The listing builds one solid part. Answer for the finished solid, in the listing's coordinates (mm). Face numbers are marked on the shaded views. Round coordinates to 2 decimals unless told otherwise and drop trailing zeros. Write each loop counter-clockwise with the first axis right and the second up, starting at its lowest first coordinate (ties: lowest second). Pieces come first, ordered by that corner, then holes.
(1) The mould has two halves that part along Y. Classify the marked faces 1, 2 and 3: +Y half, -Y half, draft (parallel to the pull), parting line (faces both ways), or undercut.
(2) A cutting plane is placed at C-C, the plane z = 0. Give the number of separate pieces and of enclosed holes in the cut face, and give its area (3 significant figures).
(3) A cutting plane is placed at D-D, the plane y = 65. Give the vertices of the cut face in (x, z), and give its area (3 significant figures).
(4) A cutting plane is placed at B-B, the plane x = -15.5. Give the vertices of the cut face in (y, z), and give its area (3 significant figures).
(5) Each of these flat-tipped pins is pushed along its axis until it touches: pin 1 Ø10 at (y, z) = (-7.5, -5) entering from -X; pin 2 Ø1.5 at (y, z) = (110.5, -10) entering from +X; pin 3 Ø5 at (y, z) = (2.5, -5.5) entering from +X. Where does it stop, or does it pass through?
(6) A cutting plane is placed at A-A, the plane x = -102. Give the vertices of the cut face in (y, z).
(7) Find the intervals of material crossed by probe 1 along Y at (x, z) = (-43.5, -7.5); probe 2 along Y at (x, z) = (-133, -2); probe 3 along Z at (x, y) = (-125, -23.55), in increasing order.
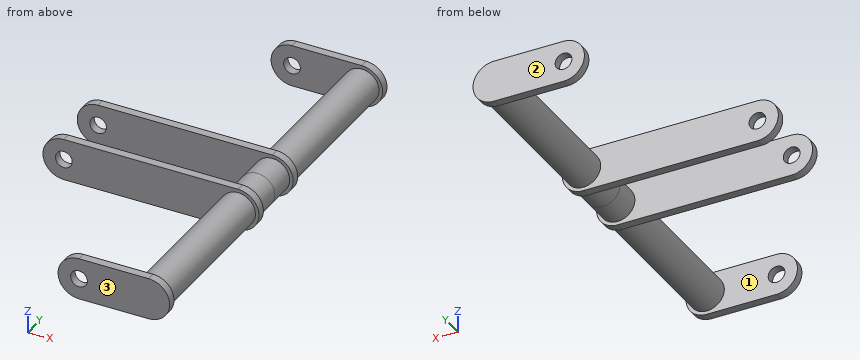
from build123d import *

# Parameters (mm, degrees)
F1_R     = 6
F1_R_2   = 12.5
F2_DEPTH = 6
F3_DEPTH = 140
F5_R     = 6
F6_DEPTH = 6


with BuildPart() as f2:
    # F1 (on offset) → F2 (new body)
    with BuildSketch(Plane.XZ.offset(140)):
        with BuildLine():
            Line((-50, -15), (0, -15))
            ThreePointArc((0, -15), (15, 0), (0, 15))
            Line((0, 15), (-50, 15))
            ThreePointArc((-50, 15), (-65, 0), (-50, -15))
        make_face()
        with Locations((-50, 0)):
            Circle(F1_R, mode=Mode.SUBTRACT)
        Circle(F1_R_2, mode=Mode.SUBTRACT)
        Circle(F1_R_2)
        Circle(F1_R, mode=Mode.SUBTRACT)
        Circle(F1_R)
    extrude(amount=F2_DEPTH)

    # F1 (on offset) → F3 (join, through all)
    with BuildSketch(Plane.XZ.offset(140)):
        Circle(F1_R_2)
        Circle(F1_R, mode=Mode.SUBTRACT)
        Circle(F1_R)
    extrude(amount=-F3_DEPTH)

    # F5 (on offset) → F6 (join)
    with BuildSketch(Plane.XZ.offset(20)):
        with BuildLine():
            Line((-125, -15), (0, -15))
            ThreePointArc((0, -15), (15, 0), (0, 15))
            Line((0, 15), (-125, 15))
            ThreePointArc((-125, 15), (-140, 0), (-125, -15))
        make_face()
        with Locations((-125, 0)):
            Circle(F5_R, mode=Mode.SUBTRACT)
    extrude(amount=F6_DEPTH)

    # F7: F2 across face


with BuildPart() as f2_1:
    add(f2.part)
    add(f2.part.mirror(Plane(origin=(0, 0, 0), x_dir=(1, 0, 0), z_dir=(0, 1, 0))))


solid = f2_1.part
Solutions:
1. face 1: undercut
1. face 2: +Y half
1. face 3: -Y half
2. separate pieces: 5
2. enclosed holes: 0
2. area: 9,230 mm2
3. outline: circle Ø25 at (0, 0)
3. area: 491 mm2
4. outline: (-146, -15) - (-140, -15) - (-140, 15) - (-146, 15) - close; (-26, -15) - (-20, -15) - (-20, 15) - (-26, 15) - close; (20, -15) - (26, -15) - (26, 15) - (20, 15) - close; (140, -15) - (146, -15) - (146, 15) - (140, 15) - close
4. area: 720 mm2
5. pin 1: stops at x = -12.5
5. pin 2: stops at x = 8.41
5. pin 3: stops at x = 12.13
6. outline: (-26, -15) - (-20, -15) - (-20, 15) - (-26, 15) - close; (20, -15) - (26, -15) - (26, 15) - (20, 15) - close
7. probe 1: y = -146 to -140, -26 to -20, 20 to 26, 140 to 146
7. probe 2: y = -26 to -20, 20 to 26
7. probe 3: z = -15 to -6, 6 to 15
